from build123d import *

# Parameters (mm, degrees)
SKETCH1_W      = 35
SKETCH1_H      = 58
SKETCH1_W_2    = 31
SKETCH1_H_2    = 54
EXTRUDE1_DEPTH = 260
FILLET1_R      = 2
SKETCH2_R      = 2.5
EXTRUDE2_DEPTH = 203.8
SKETCH3_R      = 2.5
EXTRUDE3_DEPTH = 10
EXTRUDE5_DEPTH = 26
FILLET6_R      = 2
FILLET7_R      = 2
FILLET8_R      = 2
FILLET9_R      = 2
SKETCH7_R      = 2.5
EXTRUDE6_DEPTH = 36
SKETCH8_R      = 20
SKETCH8_R_2    = 34.977592073
EXTRUDE7_DEPTH = 36


with BuildPart() as part:
    # Sketch1 → Extrude1 (new body)
    with BuildSketch(Plane.XY):
        with Locations((7.633211381, 3.238015245)):
            Rectangle(SKETCH1_W, SKETCH1_H)
        with Locations((7.633211381, 3.238015245)):
            Rectangle(SKETCH1_W_2, SKETCH1_H_2, mode=Mode.SUBTRACT)
    extrude(amount=EXTRUDE1_DEPTH)

    # Fillet1
    fillet1_edges = [part.edges().sort_by_distance(p)[0] for p in [
        (-7.866788619, 30.238015245, 130),
        (-7.866788619, -23.761984755, 130),
        (23.133211381, -23.761984755, 130),
        (23.133211381, 30.238015245, 130),
        (-9.866788619, 32.238015245, 130),
        (25.133211381, 32.238015245, 130),
        (25.133211381, -25.761984755, 130),
        (-9.866788619, -25.761984755, 130),
    ]]
    fillet(fillet1_edges, radius=FILLET1_R)

    # Sketch2 → Extrude2 (cut)
    with BuildSketch(Plane.ZY.offset(9.866788619)):
        with Locations((245, -17.761984755)):
            Circle(SKETCH2_R)
        with Locations((235, -17.761984755)):
            Circle(SKETCH2_R)
    extrude(amount=-EXTRUDE2_DEPTH, mode=Mode.SUBTRACT)

    # Sketch3 → Extrude3 (cut)
    with BuildSketch(Plane.ZY.offset(9.866788619)):
        with Locations((199, -17.761984755)):
            Circle(SKETCH3_R)
    extrude(amount=-EXTRUDE3_DEPTH, mode=Mode.SUBTRACT)

    # Sketch5 → Extrude5 (add)
    with BuildSketch(Plane(origin=(0, 0, 0), x_dir=(-1, 0, 0), z_dir=(0, 0, -1))):
        Polygon((-25.133211381, -4.739576828), (-25.133211381, -23.761984755), (-25.133211381, -25.761984755), (7.866788619, -25.761984755), (9.866788619, -25.761984755), (9.866788619, -4.739576828), (7.866788619, -4.739576828), (7.866788619, -21.761984755), (7.866788619, -23.761984755), (-23.133211381, -23.761984755), (-23.133211381, -4.739576828), align=None)
    extrude(amount=EXTRUDE5_DEPTH)

    # Fillet6
    fillet6_edges = [part.edges().sort_by_distance(p)[0] for p in [
        (25.133211381, -25.761984755, -13),
    ]]
    fillet(fillet6_edges, radius=FILLET6_R)

    # Fillet7
    fillet7_edges = [part.edges().sort_by_distance(p)[0] for p in [
        (-9.866788619, -25.761984755, -13),
    ]]
    fillet(fillet7_edges, radius=FILLET7_R)

    # Fillet8
    fillet8_edges = [part.edges().sort_by_distance(p)[0] for p in [
        (23.133211381, -23.761984755, -13),
    ]]
    fillet(fillet8_edges, radius=FILLET8_R)

    # Fillet9
    fillet9_edges = [part.edges().sort_by_distance(p)[0] for p in [
        (-7.866788619, -23.761984755, -13),
    ]]
    fillet(fillet9_edges, radius=FILLET9_R)

    # Sketch7 → Extrude6 (cut, through all)
    with BuildSketch(Plane.ZY.offset(9.866788619)):
        with Locations((-6, -17.761984755)):
            Circle(SKETCH7_R)
        with Locations((-21, -17.761984755)):
            Circle(SKETCH7_R)
    extrude(amount=-EXTRUDE6_DEPTH, mode=Mode.SUBTRACT)

    # Sketch8 → Extrude7 (cut, through all)
    with BuildSketch(Plane.ZY.offset(9.866788619)):
        with Locations((260, 9.097389033)):
            Circle(SKETCH8_R)
        with Locations((0, 30.238015245)):
            Circle(SKETCH8_R_2)
    extrude(amount=-EXTRUDE7_DEPTH, mode=Mode.SUBTRACT)


solid = part.part
Verification items for the finished model (mm, model axes). A direction names the side the tool comes from. Coordinates: 2 decimals unless noted, no trailing zeros. Write each loop counter-clockwise with the first axis right and the second up, starting at its lowest first coordinate (ties: lowest second). Pieces come first, ordered by that corner, then holes. Notation, with made-up numbers: M -38.75,-3 L -8.75,-3 A15 ccw -8.75,14 Z; hole C -40,66 d1. An arc over 180 degrees is marked long. One line per question, with ' | ' between items.
1) Sectioned sample at A-A on x = 2.5. Record the cut outline in (y, z), then the cut area to 3 significant figures.
Solutions:
outline: M -25.76,-26 L -23.76,-26 L -23.76,260 L -25.76,260 Z; M 30.24,34.98 A34.98 cw 32.24,34.92 L 32.24,260 L 30.24,260 Z | area: 1,020 mm^2
2) Material ranges on L1, parallel to X at y = -9, z = 14.5; L2, parallel to Y at x = 8, z = 151; L3, parallel to Y at x = -9, z = 245, recorded low to high.
Solutions:
L1: -9.87 to -7.87, 23.13 to 25.13 | L2: -25.76 to -23.76, 30.24 to 32.24 | L3: -25.41 to -20.26, -15.26 to -4.13, 22.33 to 31.89
3) Access from +Z, -Z, +X, -X, +Y, -Y to the whole of each face (thin tool, end or side, straight path). Record for faces 1 (the face through (-8.88, -18.72, 247.31)), 2 (the face through (23.133, 3, 119)).
Solutions:
face 1: +X, -X | face 2: +Z, -Z
4) Release check for a two-part mould opening along X. For faces 3 (the face through (-8.88, -19.98, -4.85)), 4 (the face through (-9.867, 3, 119)), 5 (the face through (-7.867, 4, 119)), 6 (the face through (7, -23.762, 119)) record: +X half, -X half, draft (parallel to the pull), parting line (faces both ways), or undercut.
Solutions:
face 3: draft | face 4: -X half | face 5: undercut | face 6: undercut
5) Sectioned sample at D-D on z = 185.5. Record the cut outline in (x, y).
Solutions:
outline: M -9.87,-23.76 A2 ccw -7.87,-25.76 L 23.13,-25.76 A2 ccw 25.13,-23.76 L 25.13,30.24 A2 ccw 23.13,32.24 L -7.87,32.24 A2 ccw -9.87,30.24 Z; hole M -7.87,-21.76 A2 ccw -5.87,-23.76 L 21.13,-23.76 A2 ccw 23.13,-21.76 L 23.13,28.24 A2 ccw 21.13,30.24 L -5.87,30.24 A2 ccw -7.87,28.24 Z
6) Sectioned sample at B-B on z = -6. Record the cut outline in (x, y).
Solutions:
outline: M -9.87,-23.76 A2 ccw -7.87,-25.76 L 23.13,-25.76 A2 ccw 25.13,-23.76 L 25.13,-20.26 L 23.13,-20.26 L 23.13,-21.76 A2 cw 21.13,-23.76 L -5.87,-23.76 A2 cw -7.87,-21.76 L -7.87,-20.26 L -9.87,-20.26 Z; M -9.87,-15.26 L -7.87,-15.26 L -7.87,-4.74 L -9.87,-4.74 Z; M 23.13,-15.26 L 25.13,-15.26 L 25.13,-4.74 L 23.13,-4.74 Z
7) Depth check by flat-ended pin: pin 1 Ø3 at (y, z) = (-17.76, 199) entering from -X; pin 2 Ø3 at (y, z) = (-17.76, 235) entering from +X; pin 3 Ø2 at (x, z) = (-8.5, -13.5) entering from +Y. Enter the tip coordinate at first touch or a pass-through.
Solutions:
pin 1: x = 23.13 | pin 2: through | pin 3: y = -4.74
8) Sectioned sample at C-C on y = 15. Record the cut outline in (x, z), then the cut area to 3 significant figures.
Solutions:
outline: M -9.87,31.48 L -7.87,31.48 L -7.87,240.89 L -9.87,240.89 Z; M 23.13,31.48 L 25.13,31.48 L 25.13,240.89 L 23.13,240.89 Z | area: 838 mm^2
